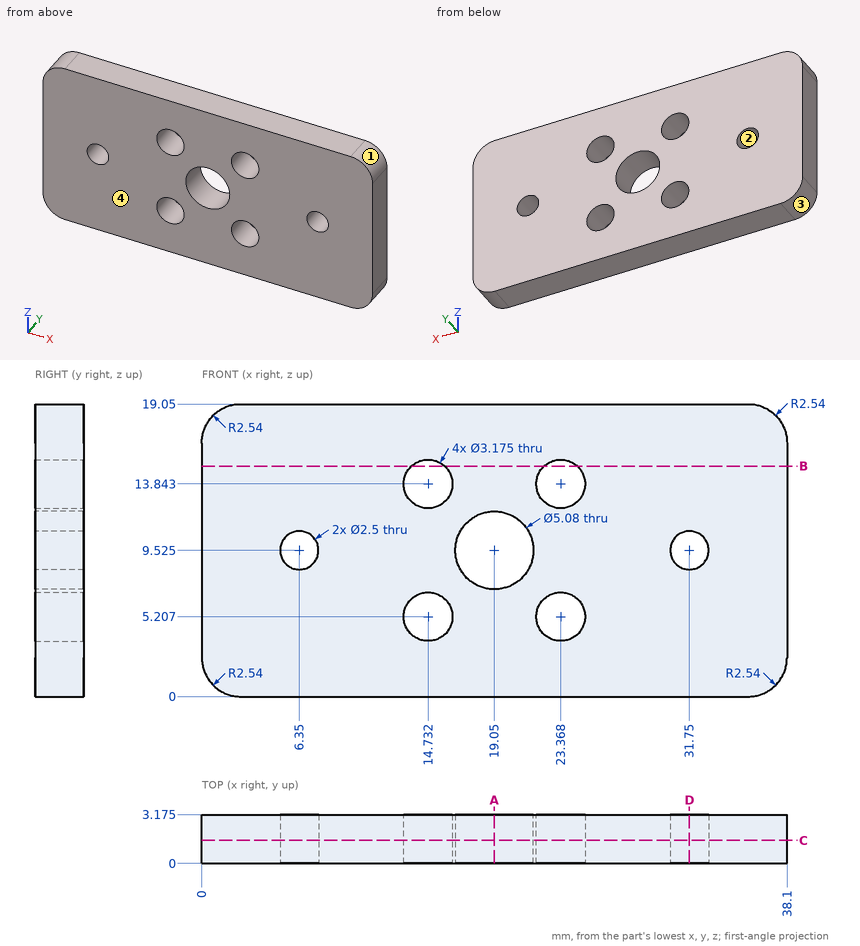
Check sheet for the drawn part. Datum: minimum x, y, z corner. Units: mm. Round coordinates to 2 decimals unless told otherwise and drop trailing zeros. Write each loop counter-clockwise with the first axis right and the second up, starting at its lowest first coordinate (ties: lowest second). Pieces come first, ordered by that corner, then holes. Notation, with made-up numbers: (-7, 20) - (44, 20) arc R16 cw to (44, 37) - close; hole circle Ø7 at (78.25, 66). An arc over 180 degrees is marked (long way). Return JSON: item names as keys, results as strings.
Q1. Cross-section at A-A (x = 19.05). Record the boundary of the cut face in (y, z) (3 decimals), then the cut area to 3 significant figures.
Returned:
{"outline": "(0, 0) - (3.175, 0) - (3.175, 6.985) - (0, 6.985) - close; (0, 12.065) - (3.175, 12.065) - (3.175, 19.05) - (0, 19.05) - close", "area": "44.4 mm²"}
Q2. Scan lines: L1, parallel to X at y = 0.4, z = 14; L2, parallel to Z at x = 6.35, y = 1 (3 decimals); L3, parallel to X at y = 0.5, z = 6.5. Record each from-to range of solid material in increasing order. Write a range as from..to.
Returned:
{"L1": "x = 0..13.15, 16.31..21.79, 24.95..38.1", "L2": "z = 0..8.275, 10.775..19.05", "L3": "x = 0..13.81, 15.65..22.45, 24.29..38.1"}
Q3. Cross-section at C-C (y = 1.5). Give the number of separate pieces and of enclosed holes in the cut face, then the cut area to 3 significant figures.
Returned:
{"separate pieces": "1", "enclosed holes": "7", "area": "659 mm²"}
Q4. Draft check along X on the marked faces 1, 2, 3 and 4. Enter one of: released by +X, released by -X, zero draft, split by the parting line, or undercut.
Returned:
{"face 1": "released by +X", "face 2": "undercut", "face 3": "released by -X", "face 4": "zero draft"}
Q5. Cross-section at B-B (z = 15). Record the boundary of the cut face in (x, y) (3 decimals), then the cut area to 3 significant figures.
Returned:
{"outline": "(0, 0) - (13.645, 0) - (13.645, 3.175) - (0, 3.175) - close; (15.819, 0) - (22.281, 0) - (22.281, 3.175) - (15.819, 3.175) - close; (24.455, 0) - (38.1, 0) - (38.1, 3.175) - (24.455, 3.175) - close", "area": "107 mm²"}
Q6. Cross-section at D-D (x = 31.75). Record the boundary of the cut face in (y, z) (3 decimals), then the cut area to 3 significant figures.
Returned:
{"outline": "(0, 0) - (3.175, 0) - (3.175, 8.275) - (0, 8.275) - close; (0, 10.775) - (3.175, 10.775) - (3.175, 19.05) - (0, 19.05) - close", "area": "52.5 mm²"}
